Here's the drawing with two shaded views (mm, measured from the low corner). I have some questions. A direction names the side the tool comes from. Give positions to 0.01 mm unless a question says otherwise; leave off trailing zeros. Loops run counter-clockwise (first coordinate to the right, second up) from the corner with the lowest first, then second, coordinate; pieces in that order, holes last. Notation, with made-up numbers: M 67,28.5 L 100,28.5 A29 ccw 100,62.5 Z; hole C -12.75,-10 d9. An arc over 180 degrees is marked long. Use a Markdown table: item, result. Add a question column.
1) Suppose I cut it at B-B on x = 30. List the corners of the cut face in (y, z) for me.
2) If I drill on line 1 along X through (y, z) = (11.3, 4); line 2 along Z through (x, y) = (30, 11.95); line 3 along X through (y, z) = (8.25, 4.5), over which ranges is the centre line in solid material (lowest first)? Write a range as [from, to].
3) Suppose I cut it at D-D on z = 1. List the corners of the cut face in (x, y) for me.
4) Will these pins go through, and if not, where does the flat tip stop? pin 1 Ø2.5 at (y, z) = (6, 2) entering from +X; pin 2 Ø1 at (y, z) = (6, 5.5) entering from -X; pin 3 Ø2 at (x, z) = (27, 6.5) entering from -Y; pin 4 Ø2 at (x, y) = (10.5, 3) entering from -Z.
5) Suppose I cut it at A-A on z = 4. List the corners of the cut face in (x, y) for me, and give its area (3 significant figures).
6) Suppose I cut it at C-C on y = 5. List the corners of the cut face in (x, z) for me.
7) Which directions (+Z, -Z, +X, -X, +Y, -Y) give clear straight access to the entire face, cutting with the end or side of a thin tool? Please do the marked faces 4, 5 and 6.
8) We'd pull the mould along Y, two halves only. Please class the marked faces 1, 2 and 3: +Y half, -Y half, draft (parallel to the pull), parting line (faces both ways), or undercut.
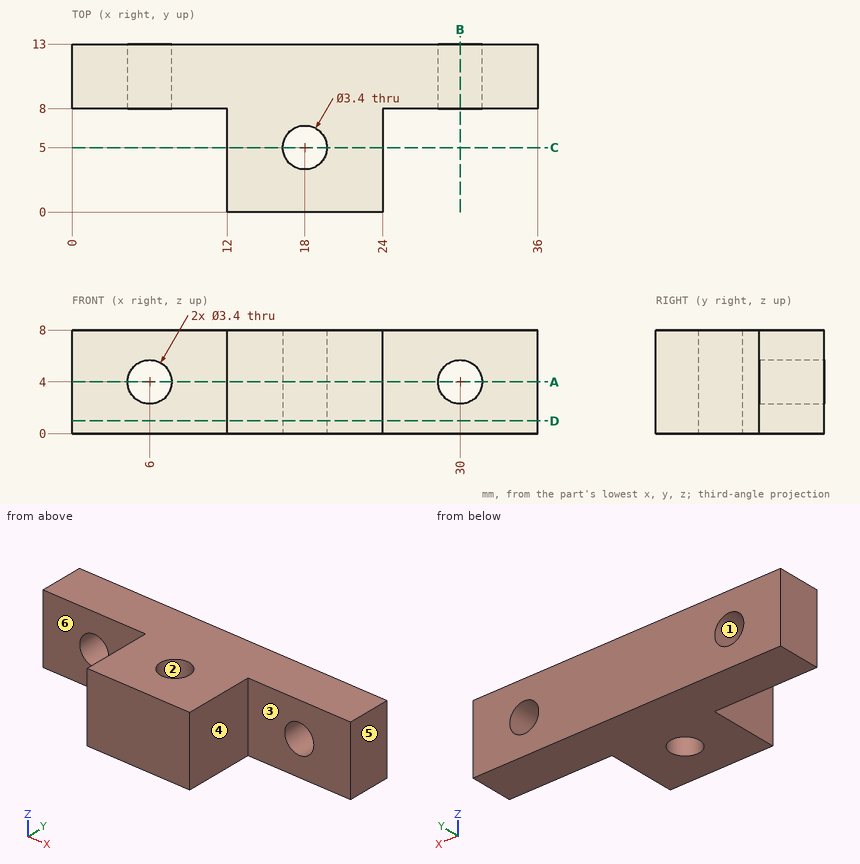
Answer block:
| question | item | result |
|---|---|---|
| 1 | outline | M 8,0 L 13,0 L 13,2.3 L 8,2.3 Z; M 8,5.7 L 13,5.7 L 13,8 L 8,8 Z |
| 2 | line 1 | x = [0, 4.3], [7.7, 28.3], [31.7, 36] |
| 2 | line 2 | z = [0, 2.3], [5.7, 8] |
| 2 | line 3 | x = [0, 4.38], [7.62, 28.38], [31.62, 36] |
| 3 | outline | M 0,8 L 12,8 L 12,0 L 24,0 L 24,8 L 36,8 L 36,13 L 0,13 Z; hole C 18,5 d3.4 |
| 4 | pin 1 | stops at x = 24 |
| 4 | pin 2 | stops at x = 12 |
| 4 | pin 3 | stops at y = 8 |
| 4 | pin 4 | passes through |
| 5 | outline | M 0,8 L 4.3,8 L 4.3,13 L 0,13 Z; M 7.7,8 L 12,8 L 12,0 L 24,0 L 24,8 L 28.3,8 L 28.3,13 L 7.7,13 Z; M 31.7,8 L 36,8 L 36,13 L 31.7,13 Z; hole C 18,5 d3.4 |
| 5 | area | 233 mm^2 |
| 6 | outline | M 12,0 L 16.3,0 L 16.3,8 L 12,8 Z; M 19.7,0 L 24,0 L 24,8 L 19.7,8 Z |
| 7 | face 4 | +Z, -Z, +X, -Y |
| 7 | face 5 | +Z, -Z, +X, +Y, -Y |
| 7 | face 6 | +Z, -Z, -X, -Y |
| 8 | face 1 | draft |
| 8 | face 2 | undercut |
| 8 | face 3 | -Y half |
